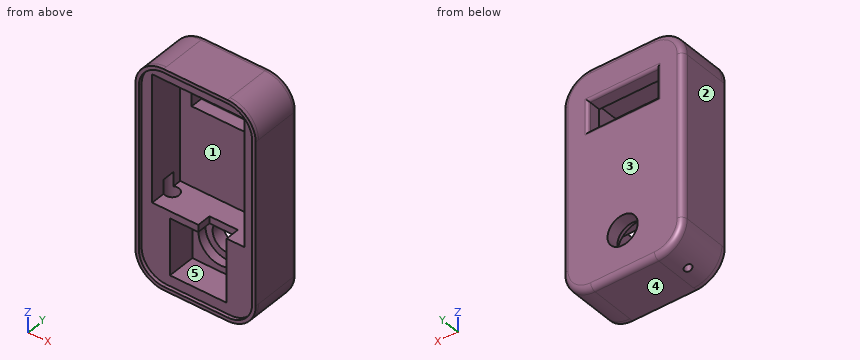
```python
from build123d import *

# Parameters (mm, degrees)
F0_W      = 107.95
F0_H      = 196.85
F1_DEPTH  = 44.45
F2_W      = 82.55
F2_H      = 114.3
F3_DEPTH  = 31.75
F4_W      = 61.9125
F4_H      = 26.9875
F5_DEPTH  = 25.4
F6_W      = 50.8
F6_H      = 50.8
F7_DEPTH  = 25.4
F8_R      = 19.84375
F9_DEPTH  = 7.9375
F10_R     = 13.49375
F11_DEPTH = 25.4
F12_R     = 25.4
F13_R     = 5.08
F14_R     = 2.54
F16_DEPTH = 3.175
F17_R     = 3.175
F18_DEPTH = 76.2
F19_R     = 6.35
F20_DEPTH = 50.8
F21_DEPTH = 12.7
F22_W     = 25.4
F22_H     = 6.35
F23_DEPTH = 12.7


with BuildPart() as f1:
    # F0 (on Front) → F1 (new body)
    with BuildSketch(Plane.XZ):
        Rectangle(F0_W, F0_H)
    extrude(amount=F1_DEPTH)

    # F2 (on face) → F3 (cut)
    with BuildSketch(Plane.XZ.offset(44.45)):
        with Locations((0, 28.575)):
            Rectangle(F2_W, F2_H)
    extrude(amount=-F3_DEPTH, mode=Mode.SUBTRACT)

    # F4 (on face) → F5 (cut)
    with BuildSketch(Plane.XZ.offset(12.7)):
        with Locations((0, 56.35625)):
            Rectangle(F4_W, F4_H)
    extrude(amount=-F5_DEPTH, mode=Mode.SUBTRACT)

    # F6 (on face) → F7 (cut)
    with BuildSketch(Plane.XZ.offset(44.45)):
        with Locations((0, -60.325)):
            Rectangle(F6_W, F6_H)
    extrude(amount=-F7_DEPTH, mode=Mode.SUBTRACT)

    # F8 (on face) → F9 (cut)
    with BuildSketch(Plane.XZ.offset(19.05)):
        with Locations((0, -60.325)):
            Circle(F8_R)
    extrude(amount=-F9_DEPTH, mode=Mode.SUBTRACT)

    # F10 (on face) → F11 (cut)
    with BuildSketch(Plane.XZ.offset(11.1125)):
        with Locations((0, -60.325)):
            Circle(F10_R)
    extrude(amount=-F11_DEPTH, mode=Mode.SUBTRACT)

    # F12
    f12_edges = [f1.edges().sort_by_distance(p)[0] for p in [
        (53.975, -22.225, 98.425),
        (53.975, -22.225, -98.425),
        (-53.975, -22.225, -98.425),
        (-53.975, -22.225, 98.425),
    ]]
    fillet(f12_edges, radius=F12_R)

    # F13
    f13_edges = [f1.edges().sort_by_distance(p)[0] for p in [
        (-53.975, 0, 0),
        (-46.535512, 0, -90.985512),
        (0, 0, -98.425),
    ]]
    fillet(f13_edges, radius=F13_R)

    # F14
    f14_edges = [f1.edges().sort_by_distance(p)[0] for p in [
        (0, 0, 69.85),
        (30.95625, 0, 56.35625),
        (0, 0, 42.8625),
        (-30.95625, 0, 56.35625),
    ]]
    fillet(f14_edges, radius=F14_R)

    # F15 (on face) → F16 (join)
    with BuildSketch(Plane.XZ.offset(44.45)):
        with BuildLine():
            ThreePointArc((53.975, 73.025), (46.5355122421, 90.9855122421), (28.575, 98.425))
            Line((28.575, 98.425), (-28.575, 98.425))
            ThreePointArc((-28.575, 98.425), (-46.5355122421, 90.9855122421), (-53.975, 73.025))
            Line((-53.975, 73.025), (-53.975, -73.025))
            ThreePointArc((-53.975, -73.025), (-46.5355122421, -90.9855122421), (-28.575, -98.425))
            Line((-28.575, -98.425), (28.575, -98.425))
            ThreePointArc((28.575, -98.425), (46.5355122421, -90.9855122421), (53.975, -73.025))
            Line((53.975, -73.025), (53.975, 73.025))
        make_face()
        with BuildLine():
            ThreePointArc((28.575, 95.25), (44.2904482119, 88.7404482119), (50.8, 73.025))
            Line((50.8, 73.025), (50.8, -73.025))
            ThreePointArc((50.8, -73.025), (44.2904482119, -88.7404482119), (28.575, -95.25))
            Line((28.575, -95.25), (-28.575, -95.25))
            ThreePointArc((-28.575, -95.25), (-44.2904482119, -88.7404482119), (-50.8, -73.025))
            Line((-50.8, -73.025), (-50.8, 73.025))
            ThreePointArc((-50.8, 73.025), (-44.2904482119, 88.7404482119), (-28.575, 95.25))
            Line((-28.575, 95.25), (28.575, 95.25))
        make_face(mode=Mode.SUBTRACT)
    extrude(amount=F16_DEPTH)

    # F17 (on face) → F18 (cut)
    with BuildSketch(Plane(origin=(0, 0, -98.425), x_dir=(1, 0, 0), z_dir=(0, 0, -1))):
        with Locations((-38.1, 25.986155495)):
            Circle(F17_R)
    extrude(amount=-F18_DEPTH, mode=Mode.SUBTRACT)

    # F19 (on face) → F20 (cut)
    with BuildSketch(Plane.XY.offset(-28.575)):
        with Locations((-38.1, -25.986155495)):
            Circle(F19_R)
    extrude(amount=-F20_DEPTH, mode=Mode.SUBTRACT)

    # F19 (on face) → F21 (cut)
    with BuildSketch(Plane.XY.offset(-28.575)):
        with Locations((-38.1, -25.986155495)):
            Circle(F19_R)
    extrude(amount=F21_DEPTH, mode=Mode.SUBTRACT)

    # F22 (on face) → F23 (cut)
    with BuildSketch(Plane.XZ.offset(44.45)):
        with Locations((12.7, -31.75)):
            Rectangle(F22_W, F22_H)
    extrude(amount=-F23_DEPTH, mode=Mode.SUBTRACT)


solid = f1.part
```
The model under review builds one solid part; all positions refer to its coordinate system, in mm. Face numbers are marked on the shaded views. A direction names the side the tool comes from. Give positions to 0.01 mm unless a question says otherwise; leave off trailing zeros. Write each loop counter-clockwise with the first axis right and the second up, starting at its lowest first coordinate (ties: lowest second). Pieces come first, ordered by that corner, then holes. Notation, with made-up numbers: (29.5, -6.75) -> (42.5, -6.75) arc R21 ccw to (42.5, 7.25) -> close; hole circle Ø10 at (16, 24). An arc over 180 degrees is marked (long way). Put each result on its own line as item: value.
(1) To check wall thickness, follow probe 1 along Z at (x, y) = (0, -16.5) (3 decimals); probe 2 along X at (y, z) = (-21, -7) (3 decimals); probe 3 along Y at (x, z) = (-38, -89). State the ranges of each line that lie inside material, in increasing order. Write a range as from..to.
Results are:
probe 1: -98.425..-80.169, -40.481..-28.575, 85.725..98.425
probe 2: -53.975..-41.275, 41.275..53.975
probe 3: -44.45..-29.16, -22.81..0
(2) Tool access review of the marked faces 1 and 2: name each direction out of +Z, -Z, +X, -X, +Y, -Y from which nothing blocks a thin tool from reaching the whole face with its end or side.
Results are:
face 1: -Y
face 2: +Z, -Z, -X, +Y, -Y
(3) We need section B-B, the plane x = 10. State how many separate pieces and enclosed holes the cut face has, and give its area (3 significant figures).
Results are:
separate pieces: 3
enclosed holes: 0
area: 2,940 mm²
(4) We need section A-A, the plane z = 50. Give the boundary of the cut face in (x, y) (3 decimals).
Results are:
outline: (-53.975, -47.625) -> (-50.8, -47.625) -> (-50.8, -44.45) -> (-41.275, -44.45) -> (-41.275, -12.7) -> (-30.956, -12.7) -> (-30.956, -2.54) arc R2.54 ccw to (-33.496, 0) -> (-48.895, 0) arc R5.08 ccw to (-53.975, -5.08) -> close; (30.956, -12.7) -> (41.275, -12.7) -> (41.275, -44.45) -> (50.8, -44.45) -> (50.8, -47.625) -> (53.975, -47.625) -> (53.975, -5.08) arc R5.08 ccw to (48.895, 0) -> (33.496, 0) arc R2.54 ccw to (30.956, -2.54) -> close
(5) For pin 1 Ø1 at (x, z) = (-13.5, 73) entering from -Y; pin 2 Ø5 at (x, z) = (7.5, -32.5) entering from -Y; pin 3 Ø1.5 at (x, z) = (-31.5, -66) entering from -Y, all flat-tipped, find the tip position at first contact; note any pin that passes through.
Results are:
pin 1: y = -12.7
pin 2: y = -31.75
pin 3: y = -44.45
(6) We need section C-C, the plane y = -40. Give the boundary of the cut face in (x, z) (3 decimals).
Results are:
outline: (-53.975, -73.025) arc R25.4 ccw to (-28.575, -98.425) -> (28.575, -98.425) arc R25.4 ccw to (53.975, -73.025) -> (53.975, 73.025) arc R25.4 ccw to (28.575, 98.425) -> (-28.575, 98.425) arc R25.4 ccw to (-53.975, 73.025) -> close; hole (-41.275, -28.575) -> (0, -28.575) -> (0, -34.925) -> (-25.4, -34.925) -> (-25.4, -85.725) -> (25.4, -85.725) -> (25.4, -28.575) -> (41.275, -28.575) -> (41.275, 85.725) -> (-41.275, 85.725) -> close
(7) The part is to be moulded in two halves that separate along Z. For the marked faces 3, 4 and 5, say which applies: pulls with the +Z half, pulls with the -Z half, needs draft (parallel to the pull), parting line crosses it, or undercut.
Results are:
face 3: needs draft
face 4: pulls with the -Z half
face 5: undercut
